```python
from build123d import *

# Parameters (mm, degrees)
CROQUIS1_R              = 4
CROQUIS1_R_2            = 20
SALIENTE_EXTRUIR1_DEPTH = 3
CROQUIS2_R              = 23
CROQUIS2_R_2            = 20
EXTRUIR_L_MINA2_DEPTH   = 30
CROQUIS3_R              = 23
SALIENTE_EXTRUIR2_DEPTH = 20
CROQUIS4_R              = 4.4
SALIENTE_EXTRUIR3_DEPTH = 20
CROQUIS6_R              = 10
SALIENTE_EXTRUIR4_DEPTH = 20


with BuildPart() as part:
    # Croquis1 → Saliente-Extruir1 (new body)
    with BuildSketch(Plane(origin=(0, 0, 0), x_dir=(0, 0, -1), z_dir=(1, 0, 0))):
        with BuildLine():
            ThreePointArc((6.186895244, 41.036231884), (0, 43.5), (-6.186895244, 41.036231884))
            ThreePointArc((-6.186895244, 41.036231884), (-29.344931419, 29.344931419), (-41.036231884, 6.186895244))
            ThreePointArc((-41.036231884, 6.186895244), (-43.5, 0), (-41.036231884, -6.186895244))
            ThreePointArc((-41.036231884, -6.186895244), (-29.344931419, -29.344931419), (-6.186895244, -41.036231884))
            ThreePointArc((-6.186895244, -41.036231884), (0, -43.5), (6.186895244, -41.036231884))
            ThreePointArc((6.186895244, -41.036231884), (29.344931419, -29.344931419), (41.036231884, -6.186895244))
            ThreePointArc((41.036231884, -6.186895244), (43.5, 0), (41.036231884, 6.186895244))
            ThreePointArc((41.036231884, 6.186895244), (29.344931419, 29.344931419), (6.186895244, 41.036231884))
        make_face()
        with Locations((0, -34.5)):
            Circle(CROQUIS1_R, mode=Mode.SUBTRACT)
        with Locations((-34.5, 0)):
            Circle(CROQUIS1_R, mode=Mode.SUBTRACT)
        Circle(CROQUIS1_R_2, mode=Mode.SUBTRACT)
        with Locations((0, 34.5)):
            Circle(CROQUIS1_R, mode=Mode.SUBTRACT)
        with Locations((34.5, 0)):
            Circle(CROQUIS1_R, mode=Mode.SUBTRACT)
    extrude(amount=SALIENTE_EXTRUIR1_DEPTH)

    # Croquis2 → Extruir-Lámina2 (add)
    with BuildSketch(Plane(origin=(3, 0, 0), x_dir=(0, 0, -1), z_dir=(1, 0, 0))):
        Circle(CROQUIS2_R)
        Circle(CROQUIS2_R_2, mode=Mode.SUBTRACT)
    extrude(amount=EXTRUIR_L_MINA2_DEPTH)

    # Croquis3 → Saliente-Extruir2 (add)
    with BuildSketch(Plane(origin=(33, 0, 0), x_dir=(0, 0, -1), z_dir=(1, 0, 0))):
        Circle(CROQUIS3_R)
    extrude(amount=SALIENTE_EXTRUIR2_DEPTH)

    # Croquis4 → Saliente-Extruir3 (add)
    with BuildSketch(Plane.ZY.offset(-33)):
        with Locations(Location((0, 0, 0), (0, 0, 180))):
            Circle(CROQUIS4_R)
    extrude(amount=SALIENTE_EXTRUIR3_DEPTH)

    # Croquis5 → Revolución1 (revolve)
    with BuildSketch(Plane(origin=(0, 0, 0), x_dir=(1, 0, 0), z_dir=(0, 1, 0))):
        Polygon((48, -23), (3, -29), (3, -23), align=None)
    revolve(axis=Axis((-12.262234232, 0, 0), (1, 0, 0)))

    # Croquis6 → Saliente-Extruir4 (add)
    with BuildSketch(Plane(origin=(53, 0, 0), x_dir=(0, 0, -1), z_dir=(1, 0, 0))):
        Circle(CROQUIS6_R)
        with BuildLine():
            Line((-1.307669683, 2.7), (1.307669683, 2.7))
            ThreePointArc((1.307669683, 2.7), (0, -3), (-1.307669683, 2.7))
        make_face(mode=Mode.SUBTRACT)
    extrude(amount=SALIENTE_EXTRUIR4_DEPTH)


solid = part.part
```
Input: part model. Units: mm. Frame: model coordinates. A direction names the side the tool comes from. Give positions to 0.01 mm unless a question says otherwise; leave off trailing zeros. Order: outer loops, then holes, each group sorted by start corner. A loop starts at its lowest first (then second) coordinate and runs counter-clockwise, first axis right, second up. Notation, with made-up numbers: (12.25, 4.25) -> (68.25, 4.25) arc R22 cw to (68.25, 13.25) -> close; hole circle Ø2 at (64.5, 17.25). An arc over 180 degrees is marked (long way). Write each question's results on one line, items separated by ' | '. Start each with the question number.
Item 1: Cut plane A-A on z = 0. Give the number of separate pieces and of enclosed holes in the cut face, then the cut area to 4 significant figures.
Item 2: Contact query for flat-ended pins moving along their axis: P1, Ø1.5, axis at x = 14.5, z = 20.5, coming from the -Y side; P2, Ø3, axis at y = 0.5, z = -1, coming from the +X side; P3, Ø5.5, axis at y = 0, z = 0, coming from the -X side; P4, Ø12, axis at x = 34.5, y = 31.5, coming from the +Z side. Output: stop coordinate, or through.
Item 3: Line query: line 1 (Z direction, x = 30, y = -4); line 2 (Z direction, x = 24, y = 3.5); line 3 (X direction, y = -9, z = -6). Output: solid intervals per line, ascending.
Item 4: Cut plane C-C on z = -34.5. Return the cut outline in (x, y).
Item 5: Mould query, pull axis Y, two halves, no side actions, for faces 4 (the flat face through (53, -5, -10)), 5 (the flat face through (63, 2.7, 0)), 6 (the cylindrical face through (1.479, 29.083, -29.605)). Classes: pulls with the +Y half, pulls with the -Y half, needs draft (parallel to the pull), parting line crosses it, or undercut.
Item 6: Set-up query: faces 1 (the cylindrical face through (1.5, 43.5, -0.1)), 2 (the flat face through (33, 5, 0)), 3 (the flat face through (53, 0, 0)). Return all of +Z, -Z, +X, -X, +Y, -Y with unobstructed straight access to the full face (end or side cutting, diameter ignored); none if empty.
Established:
1) separate pieces: 3 | enclosed holes: 0 | area: 1,925 mm^2
2) P1: y = -19.1 | P2: x = 53 | P3: x = 13 | P4: through
3) line 1: -25.08 to -19.6, -1.83 to 1.83, 19.6 to 25.08 | line 2: -25.97 to -19.69, -2.67 to 2.67, 19.69 to 25.97 | line 3: 33 to 53
4) outline: (0, -23.07) -> (3, -23.07) -> (3, -4) -> (0, -4) -> close; (0, 4) -> (3, 4) -> (3, 23.07) -> (0, 23.07) -> close
5) face 4: needs draft | face 5: undercut | face 6: pulls with the +Y half
6) face 1: +X, -X, +Y | face 2: -X | face 3: +X
